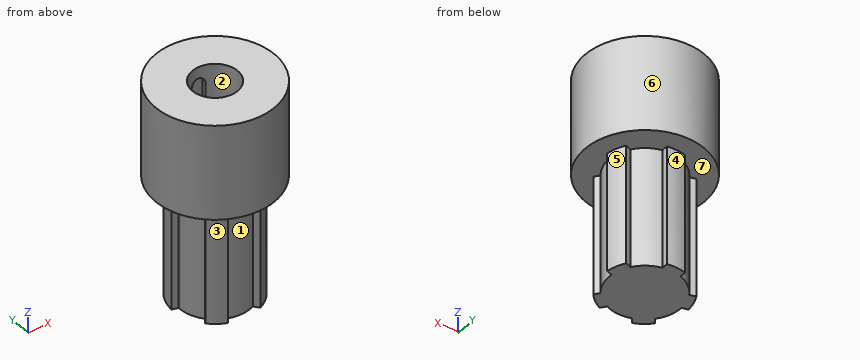
from build123d import *

# Parameters (mm, degrees)
SKETCH1_R           = 25
BOSS_EXTRUDE1_DEPTH = 90
SKETCH2_R           = 25
CUT_EXTRUDE2_DEPTH  = 50
CUT_EXTRUDE4_DEPTH  = 50
SKETCH3_R           = 9.5
CUT_EXTRUDE5_DEPTH  = 29.2
CUT_EXTRUDE6_DEPTH  = 4


with BuildPart() as part:
    # Sketch1 → Boss-Extrude1 (new body)
    with BuildSketch(Plane.XY):
        with Locations(Location((0, 0, 0), (0, 0, 180))):
            Circle(SKETCH1_R)
    extrude(amount=BOSS_EXTRUDE1_DEPTH)

    # Sketch2 → Cut-Extrude2 (cut)
    with BuildSketch(Plane(origin=(0, 0, 0), x_dir=(-1, 0, 0), z_dir=(0, 0, -1))):
        Circle(SKETCH2_R)
        with BuildLine():
            ThreePointArc((3.88, 17.064454284), (10.286241915, 14.157797402), (15.030274505, 8.963305657))
            ThreePointArc((15.030274505, 8.963305657), (16.643489035, 5.407797402), (17.428246382, 1.58310709))
            ThreePointArc((17.428246382, 1.58310709), (17.482052392, 0.792366178), (17.5, 0))
            ThreePointArc((17.5, 0), (16.381565231, -6.155836303), (13.169220505, -11.524826736))
            ThreePointArc((13.169220505, -11.524826736), (10.286241915, -14.157797402), (6.891248628, -16.086040294))
            ThreePointArc((6.891248628, -16.086040294), (0, -17.5), (-6.891248628, -16.086040294))
            ThreePointArc((-6.891248628, -16.086040294), (-10.286241915, -14.157797402), (-13.169220505, -11.524826736))
            ThreePointArc((-13.169220505, -11.524826736), (-16.643489035, -5.407797402), (-17.428246382, 1.58310709))
            ThreePointArc((-17.428246382, 1.58310709), (-16.643489035, 5.407797402), (-15.030274505, 8.963305657))
            ThreePointArc((-15.030274505, 8.963305657), (-10.286241915, 14.157797402), (-3.88, 17.064454284))
            ThreePointArc((-3.88, 17.064454284), (0, 17.5), (3.88, 17.064454284))
        make_face(mode=Mode.SUBTRACT)
    extrude(amount=-CUT_EXTRUDE2_DEPTH, mode=Mode.SUBTRACT)

    # Sketch2_3 → Cut-Extrude4 (cut)
    with BuildSketch(Plane(origin=(0, 0, 0), x_dir=(-1, 0, 0), z_dir=(0, 0, -1))):
        with BuildLine():
            Line((-3.88, 14.489499646), (-3.88, 17.064454284))
            ThreePointArc((-3.88, 17.064454284), (-10.286241915, 14.157797402), (-15.030274505, 8.963305657))
            Line((-15.030274505, 8.963305657), (-12.581347118, 8.167600914))
            ThreePointArc((-12.581347118, 8.167600914), (-8.816778784, 12.135254916), (-3.88, 14.489499646))
        make_face()
        with BuildLine():
            ThreePointArc((3.88, 14.489499646), (8.816778784, 12.135254916), (12.581347118, 8.167600914))
            Line((12.581347118, 8.167600914), (15.030274505, 8.963305657))
            ThreePointArc((15.030274505, 8.963305657), (10.286241915, 14.157797402), (3.88, 17.064454284))
            Line((3.88, 17.064454284), (3.88, 14.489499646))
        make_face()
        with BuildLine():
            Line((17.428246382, 1.58310709), (14.979318995, 0.787402347))
            ThreePointArc((14.979318995, 0.787402347), (14.994828857, 0.393836946), (15, 0))
            ThreePointArc((15, 0), (14.139227386, -5.008218139), (11.655700143, -9.441644675))
            Line((11.655700143, -9.441644675), (13.169220505, -11.524826736))
            ThreePointArc((13.169220505, -11.524826736), (16.381565231, -6.155836303), (17.5, 0))
            ThreePointArc((17.5, 0), (17.482052392, 0.792366178), (17.428246382, 1.58310709))
        make_face()
        with BuildLine():
            Line((6.891248628, -16.086040294), (5.377728267, -14.002858233))
            ThreePointArc((5.377728267, -14.002858233), (0, -15), (-5.377728267, -14.002858233))
            Line((-5.377728267, -14.002858233), (-6.891248628, -16.086040294))
            ThreePointArc((-6.891248628, -16.086040294), (0, -17.5), (6.891248628, -16.086040294))
        make_face()
        with BuildLine():
            Line((-14.979318995, 0.787402347), (-17.428246382, 1.58310709))
            ThreePointArc((-17.428246382, 1.58310709), (-16.643489035, -5.407797402), (-13.169220505, -11.524826736))
            Line((-13.169220505, -11.524826736), (-11.655700143, -9.441644675))
            ThreePointArc((-11.655700143, -9.441644675), (-14.265847744, -4.635254916), (-14.979318995, 0.787402347))
        make_face()
    extrude(amount=-CUT_EXTRUDE4_DEPTH, mode=Mode.SUBTRACT)

    # Sketch3 → Cut-Extrude5 (cut)
    with BuildSketch(Plane.XY.offset(90)):
        Circle(SKETCH3_R)
    extrude(amount=-CUT_EXTRUDE5_DEPTH, mode=Mode.SUBTRACT)

    # Sketch5 → Cut-Extrude6 (cut)
    with BuildSketch(Plane(origin=(0, 6.68, 0), x_dir=(1, 0, 0), z_dir=(0, 1, 0))):
        with BuildLine():
            Line((-3, -82.2), (-3, -57.2))
            ThreePointArc((-3, -57.2), (0, -54.2), (3, -57.2))
            Line((3, -57.2), (3, -82.2))
            ThreePointArc((3, -82.2), (0, -85.2), (-3, -82.2))
        make_face()
    extrude(amount=CUT_EXTRUDE6_DEPTH, mode=Mode.SUBTRACT)


solid = part.part
Here's how the part is built. I have some questions about the finished solid (model axes, mm). Face numbers are marked on the shaded views. A direction names the side the tool comes from. Coordinates: 2 decimals unless noted, no trailing zeros. Order: outer loops, then holes, each group sorted by start corner. A loop starts at its lowest first (then second) coordinate and runs counter-clockwise, first axis right, second up. Notation, with made-up numbers: M -40,49 L 1,49 A24 cw 1,73 Z; hole C 64,-36 d6. An arc over 180 degrees is marked long. Answer as CSV lines item,"result".
Item 1: For pin 1 (2 mm diameter, centred on x = 9, z = 13, fed in from -Y); pin 2 (1.5 mm diameter, centred on y = -7.5, z = 50, fed in from -X); pin 3 (9.5 mm diameter, centred on x = 4, y = 3.5, fed in from +Z); pin 4 (3 mm diameter, centred on y = 15, z = 28, fed in from +X), each with a flat end and sliding along its axis, tell me the tip position at first contact or that it passes through.
Results found:
pin 1,"y = -15.56"
pin 2,"x = -24.07"
pin 3,"z = 90"
pin 4,"x = 6.54"
Item 2: We'd pull the mould along X, two halves only. Please class the marked faces 1, 2, 3 and 4: +X half, -X half, draft (parallel to the pull), parting line (faces both ways), or undercut.
Results found:
face 1,"undercut"
face 2,"undercut"
face 3,"-X half"
face 4,"parting line"
Item 3: Imagine slicing it at A-A on z = 64. Write out the boundary of the cut face in (x, y).
Results found:
outline,"C 0,0 d50; hole M -3,9.01 A9.5 ccw long 3,9.01 L 3,10.68 L -3,10.68 Z"
Item 4: If I drill on line 1 (Y direction, x = 0, z = 76.5); line 2 (Z direction, x = -5, y = -15); line 3 (X direction, y = 0, z = 76), over which ranges is the centre line in solid material (lowest first)?
Results found:
line 1,"-25 to -9.5, 10.68 to 25"
line 2,"50 to 90"
line 3,"-25 to -9.5, 9.5 to 25"
Item 5: Imagine slicing it at D-D on z = 8. Write out the boundary of the cut face in (x, y), plus the area to 3 significant figures.
Results found:
outline,"M -17.43,1.58 L -14.98,0.79 A15 ccw -15,0 A15 ccw -11.66,-9.44 L -13.17,-11.52 A17.5 ccw -6.89,-16.09 L -5.38,-14 A15 ccw 5.38,-14 L 6.89,-16.09 A17.5 ccw 13.17,-11.52 L 11.66,-9.44 A15 ccw 14.98,0.79 L 17.43,1.58 A17.5 ccw 15.03,8.96 L 12.58,8.17 A15 ccw 3.88,14.49 L 3.88,17.06 A17.5 ccw -3.88,17.06 L -3.88,14.49 A15 ccw -12.58,8.17 L -15.03,8.96 A17.5 ccw Z"
area,"805 mm2"
Item 6: On a 3-axis mill with a long thin cutter (end or side, diameter ignored), from which of +Z, -Z, +X, -X, +Y, -Y can I reach the whole of each face in a straight line? I mean the marked faces 5, 6 and 7. Say none if no direction works.
Results found:
face 5,"-Z, +X, +Y"
face 6,"+Z, -Z"
face 7,"-Z"
Item 7: Imagine slicing it at B-B on x = 0. Write out the boundary of the cut face in (y, z).
Results found:
outline,"M -25,50 L -15,50 L -15,0 L 17.5,0 L 17.5,50 L 25,50 L 25,90 L 9.5,90 L 9.5,85.2 L 10.68,85.2 L 10.68,54.2 L 6.68,54.2 L 6.68,60.8 L -9.5,60.8 L -9.5,90 L -25,90 Z"
Item 8: Imagine slicing it at C-C on y = -6. Write out the boundary of the cut face in (x, z), plus the area to 3 significant figures.
Results found:
outline,"M -24.27,50 L -13.75,50 L -13.75,0 L 13.75,0 L 13.75,50 L 24.27,50 L 24.27,90 L 7.37,90 L 7.37,60.8 L -7.37,60.8 L -7.37,90 L -24.27,90 Z"
area,"2,890 mm2"
